```python
from build123d import *

# Parameters (mm, degrees)
SKETCH2_R           = 1.75
SKETCH2_R_2         = 7.5
FLANGE_DEPTH        = 5
SKETCH3_R           = 8.5
O_RING_SEAT_DEPTH   = 0.5
SKETCH5_R           = 1
OUTLET_DEPTH        = 38.107950631
BOSS_EXTRUDE2_REACH = 55.944
SKETCH6_R           = 2.5
SKETCH6_R_2         = 1
CIRPATTERN1_COUNT   = 2


with BuildPart() as part:
    # Sketch2 → Flange (new body)
    with BuildSketch(Plane(origin=(0, 0, 0), x_dir=(0, 0, -1), z_dir=(1, 0, 0))):
        with BuildLine():
            Line((-6.717514421, 6.717514421), (-2.92760615, 23.655074219))
            ThreePointArc((-2.92760615, 23.655074219), (0, 26), (2.92760615, 23.655074219))
            Line((2.92760615, 23.655074219), (6.717514421, 6.717514421))
            Line((6.717514421, 6.717514421), (23.655074219, 2.92760615))
            ThreePointArc((23.655074219, 2.92760615), (26, 0), (23.655074219, -2.92760615))
            Line((23.655074219, -2.92760615), (6.717514421, -6.717514421))
            Line((6.717514421, -6.717514421), (2.92760615, -23.655074219))
            ThreePointArc((2.92760615, -23.655074219), (0, -26), (-2.92760615, -23.655074219))
            Line((-2.92760615, -23.655074219), (-6.717514421, -6.717514421))
            Line((-6.717514421, -6.717514421), (-23.655074219, -2.92760615))
            ThreePointArc((-23.655074219, -2.92760615), (-26, 0), (-23.655074219, 2.92760615))
            Line((-23.655074219, 2.92760615), (-6.717514421, 6.717514421))
        make_face()
        with Locations((0, 23)):
            Circle(SKETCH2_R, mode=Mode.SUBTRACT)
        with Locations((23, 0)):
            Circle(SKETCH2_R, mode=Mode.SUBTRACT)
        with Locations((0, -23)):
            Circle(SKETCH2_R, mode=Mode.SUBTRACT)
        with Locations((-23, 0)):
            Circle(SKETCH2_R, mode=Mode.SUBTRACT)
        Circle(SKETCH2_R_2, mode=Mode.SUBTRACT)
    extrude(amount=FLANGE_DEPTH)

    # Sketch3 → O-Ring Seat (cut)
    with BuildSketch(Plane(origin=(5, 0, 0), x_dir=(0, 0, -1), z_dir=(1, 0, 0))):
        Circle(SKETCH3_R)
    o_ring_seat = extrude(amount=-O_RING_SEAT_DEPTH, mode=Mode.SUBTRACT)

    # Mirror1: O-Ring Seat across plane
    add(o_ring_seat.mirror(Plane(origin=(2.5, 0, 0), x_dir=(0, 0, 1), z_dir=(1, 0, 0))), mode=Mode.SUBTRACT)

    # Sketch5 → Outlet (cut, through all)
    with BuildSketch(Plane(origin=(0, 0, 0), x_dir=(1, 0, 0), z_dir=(0, 1, 0))):
        with Locations(Location((2.5, 6.5, 0), (0, 0, 90))):
            Circle(SKETCH5_R)
    outlet = extrude(amount=OUTLET_DEPTH, mode=Mode.SUBTRACT)

    # Sketch6 → Boss-Extrude2 (add, up to next)
    with BuildSketch(Plane(origin=(0, 21, 0), x_dir=(1, 0, 0), z_dir=(0, 1, 0)), mode=Mode.PRIVATE) as boss_extrude2_sk1:
        with Locations(Location((2.5, 6.5, 0), (0, 0, 270))):
            Circle(SKETCH6_R)
        with Locations(Location((2.5, 6.5, 0), (0, 0, 90))):
            Circle(SKETCH6_R_2, mode=Mode.SUBTRACT)
    boss_extrude2_tool1 = extrude(boss_extrude2_sk1.sketch, amount=-BOSS_EXTRUDE2_REACH, mode=Mode.PRIVATE) - part.part
    boss_extrude2 = boss_extrude2_tool1.solids().sort_by_distance((2.5, 21, -8.929289))[0]
    add(boss_extrude2)

    # Sketch8 → Revolve1 (revolve)
    with BuildSketch(Plane(origin=(2.5, 0, 0), x_dir=(0, 0, -1), z_dir=(1, 0, 0))):
        Polygon((5, 21), (5, 22), (4.5, 22), (5, 24), (4.5, 24), (5, 26), (4.5, 26), (5, 28), (5.5, 28), (5.5, 21), align=None)
    revolve1 = revolve(axis=Axis((2.5, 26, -6.5), (0, -1, 0)))

    # CirPattern1: Outlet, Boss-Extrude2, Revolve1 ×2 about axis
    cirpattern1_axis = Axis((0.5, 0, 0), (-1, 0, 0))
    add([outlet.rotate(cirpattern1_axis, i * 360 / CIRPATTERN1_COUNT) for i in range(1, CIRPATTERN1_COUNT)], mode=Mode.SUBTRACT)
    add([boss_extrude2.rotate(cirpattern1_axis, i * 360 / CIRPATTERN1_COUNT) for i in range(1, CIRPATTERN1_COUNT)])
    add([revolve1.rotate(cirpattern1_axis, i * 360 / CIRPATTERN1_COUNT) for i in range(1, CIRPATTERN1_COUNT)])


solid = part.part
```
Check sheet for the modelled part. Datum: model origin and axes. Units: mm. A direction names the side the tool comes from. Coordinates: 2 decimals unless noted, no trailing zeros. Write each loop counter-clockwise with the first axis right and the second up, starting at its lowest first coordinate (ties: lowest second). Pieces come first, ordered by that corner, then holes. Notation, with made-up numbers: M 11,36.5 L 67,36.5 A22 cw 67,70.5 Z; hole C 53,43.5 d8. An arc over 180 degrees is marked long. Write item = value, one per line. Start each with the question number.
1. Tool access check on faces 4 (the cylindrical face through (4.754, 7.167, -4.57)), 5 (the cylindrical face through (1.502, -16.915, 6.566)), 6 (the cylindrical face through (0.246, 7.167, -4.57)). Record the directions out of +Z, -Z, +X, -X, +Y, -Y that give a thin tool (end or side, any length) a straight path to the whole face; none if there is none.
2. Mould release check, pull along Y, two halves, no side actions. Record for faces 1 (the flat face through (2.46, -4.85, 15.07)), 2 (the cylindrical face through (1.502, 16.915, -6.566)), 3 (the flat face through (4.5, -8, 0)): pulls with the +Y half, pulls with the -Y half, needs draft (parallel to the pull), parting line crosses it, or undercut.
3. Thickness scan on probe 1 along Y at (x, z) = (2.85, 0); probe 2 along Y at (x, z) = (0.2, 0); probe 3 along Z at (x, y) = (2.35, -25). Record the ranges inside material, lowest first.
4. Go/stop test with flat-tipped pins: pin 1 (5 mm diameter, centred on y = -3, z = -3, fed in from +X); pin 2 (1 mm diameter, centred on x = 4, y = -2.5, fed in from -Z); pin 3 (1.5 mm diameter, centred on x = 3.5, z = 15.5, fed in from -Y); pin 4 (1.5 mm diameter, centred on x = 2.5, z = -2.5, fed in from +Y). Record where each tip stops, or that it passes through.
5. Sectioned sample at C-C (z = -23). Record the cut outline in (x, y).
6. Sectioned sample at D-D (y = 10.5). Record the cut outline in (x, z), then the cut area to 3 significant figures.
7. Sectioned sample at B-B (y = -23). Record the cut outline in (x, z), then the cut area to 3 significant figures.
8. Sectioned sample at A-A (z = 0). Record the cut outline in (x, y), then the cut area to 3 significant figures.
The answers:
q1.face_4 = +X
q1.face_5 = -Y
q1.face_6 = -X
q2.face_1 = pulls with the -Y half
q2.face_2 = needs draft
q2.face_3 = undercut
q3.probe_1 = -26 to -24.75, -21.25 to -7.5, 7.5 to 21.25, 24.75 to 26
q3.probe_2 = -26 to -24.75, -21.25 to -8.5, 8.5 to 21.25, 24.75 to 26
q3.probe_3 = -2.24 to 2.24, 4.76 to 5.51, 7.49 to 8.24
q4.pin_1 = through
q4.pin_2 = -25.24
q4.pin_3 = -4.92
q4.pin_4 = 25.44
q5.outline = M 0,-3.07 L 5,-3.07 L 5,-1.75 L 0,-1.75 Z; M 0,1.75 L 5,1.75 L 5,3.07 L 0,3.07 Z
q6.outline = M 0,-5.87 L 0.08,-5.87 A2.5 ccw long 4.92,-5.87 L 5,-5.87 L 5,5.87 L 0,5.87 Z; hole C 2.5,-6.5 d2
q6.area = 68.5 mm²
q7.outline = M 0,-3.07 L 5,-3.07 L 5,-1.75 L 0,-1.75 Z; M 0,1.75 L 5,1.75 L 5,3.07 L 0,3.07 Z; C 2.5,6.5 d3.5; hole C 2.5,6.5 d2
q7.area = 19.7 mm²
q8.outline = M 0,-26 L 5,-26 L 5,-24.75 L 0,-24.75 Z; M 0,-21.25 L 5,-21.25 L 5,-8.5 L 4.5,-8.5 L 4.5,-7.5 L 0.5,-7.5 L 0.5,-8.5 L 0,-8.5 Z; M 0,8.5 L 0.5,8.5 L 0.5,7.5 L 4.5,7.5 L 4.5,8.5 L 5,8.5 L 5,21.25 L 0,21.25 Z; M 0,24.75 L 5,24.75 L 5,26 L 0,26 Z
q8.area = 148 mm²
